For this review, take the finished solid that the model builds, in its own axes (mm). A direction names the side the tool comes from. Coordinates: 2 decimals unless noted, no trailing zeros. Write each loop counter-clockwise with the first axis right and the second up, starting at its lowest first coordinate (ties: lowest second). Pieces come first, ordered by that corner, then holes. Notation, with made-up numbers: M 19,31.25 L 50,31.25 A17 ccw 50,52.25 Z; hole C -3,-5.5 d2. An arc over 180 degrees is marked long. One line per question, with ' | ' between items.
from build123d import *

# Parameters (mm, degrees)
BOSS_EXTRUDE1_DEPTH = 10
BOSS_EXTRUDE2_DEPTH = 10
SKETCH3_R           = 18.5
CUT_EXTRUDE1_DEPTH  = 7
SKETCH4_R           = 14
CUT_EXTRUDE2_DEPTH  = 181.671916356
SKETCH5_R           = 3.5
CUT_EXTRUDE3_DEPTH  = 181.671916356
SKETCH6_R           = 8
CUT_EXTRUDE4_DEPTH  = 5
CUT_EXTRUDE5_DEPTH  = 4


with BuildPart() as part:
    # Sketch1 → Boss-Extrude1 (new body)
    with BuildSketch(Plane(origin=(0, 0, 0), x_dir=(1, 0, 0), z_dir=(0, 1, 0))):
        with BuildLine():
            Line((-50.126401057, 19.839201524), (-7.169705454, -10.239400554))
            ThreePointArc((-7.169705454, -10.239400554), (0, -12.5), (7.169705454, -10.239400554))
            Line((7.169705454, -10.239400554), (50.126401057, 19.839201524))
            ThreePointArc((50.126401057, 19.839201524), (54.194564303, 26.060188175), (52.845996063, 33.369907103))
            ThreePointArc((52.845996063, 33.369907103), (0, 62.5), (-52.845996063, 33.369907103))
            ThreePointArc((-52.845996063, 33.369907103), (-54.194564303, 26.060188175), (-50.126401057, 19.839201524))
        make_face()
    extrude(amount=BOSS_EXTRUDE1_DEPTH)

    # Sketch2 → Boss-Extrude2 (add)
    with BuildSketch(Plane(origin=(0, 0, 0), x_dir=(1, 0, 0), z_dir=(0, 1, 0))):
        with BuildLine():
            Line((-22, 0.144883481), (-22, -150))
            ThreePointArc((-22, -150), (0, -172), (22, -150))
            Line((22, -150), (22, 0.144883481))
            Line((22, 0.144883481), (7.169705454, -10.239400554))
            ThreePointArc((7.169705454, -10.239400554), (0, -12.5), (-7.169705454, -10.239400554))
            Line((-7.169705454, -10.239400554), (-22, 0.144883481))
        make_face()
    extrude(amount=BOSS_EXTRUDE2_DEPTH)

    # Sketch3 → Cut-Extrude1 (cut)
    with BuildSketch(Plane(origin=(0, 10, 0), x_dir=(1, 0, 0), z_dir=(0, 1, 0))):
        with Locations(Location((0, 0, 0), (0, 0, 270))):
            Circle(SKETCH3_R)
    extrude(amount=-CUT_EXTRUDE1_DEPTH, mode=Mode.SUBTRACT)

    # Sketch4 → Cut-Extrude2 (cut, through all)
    with BuildSketch(Plane(origin=(0, 10, 0), x_dir=(1, 0, 0), z_dir=(0, 1, 0))):
        with Locations(Location((0, 0, 0), (0, 0, 270))):
            Circle(SKETCH4_R)
    extrude(amount=-CUT_EXTRUDE2_DEPTH, mode=Mode.SUBTRACT)

    # Sketch5 → Cut-Extrude3 (cut, through all)
    with BuildSketch(Plane(origin=(0, 10, 0), x_dir=(1, 0, 0), z_dir=(0, 1, 0))):
        with Locations(Location((0, -150, 0), (0, 0, 270))):
            Circle(SKETCH5_R)
    extrude(amount=-CUT_EXTRUDE3_DEPTH, mode=Mode.SUBTRACT)

    # Sketch6 → Cut-Extrude4 (cut)
    with BuildSketch(Plane.XZ):
        with Locations(Location((0, 150, 0), (0, 0, 270))):
            Circle(SKETCH6_R)
    extrude(amount=-CUT_EXTRUDE4_DEPTH, mode=Mode.SUBTRACT)

    # Sketch7 → Cut-Extrude5 (cut)
    with BuildSketch(Plane(origin=(0, 10, 0), x_dir=(1, 0, 0), z_dir=(0, 1, 0))):
        Polygon((4.618802154, -150), (2.309401077, -146), (-2.309401077, -146), (-4.618802154, -150), (-2.309401077, -154), (2.309401077, -154), align=None)
    extrude(amount=-CUT_EXTRUDE5_DEPTH, mode=Mode.SUBTRACT)


solid = part.part
1) We need section C-C on z = 110.5. State the section outline as (x, y) points, then the cut area to 3 significant figures.
Responses:
outline: M -22,0 L 22,0 L 22,10 L -22,10 Z | area: 440 mm^2
2) We need section A-A on x = 0. State the section outline as (y, z) points, then the cut area to 3 significant figures.
Responses:
outline: M 0,-62.5 L 10,-62.5 L 10,-18.5 L 3,-18.5 L 3,-14 L 0,-14 Z; M 0,14 L 3,14 L 3,18.5 L 10,18.5 L 10,146 L 6,146 L 6,146.5 L 5,146.5 L 5,142 L 0,142 Z; M 0,158 L 5,158 L 5,153.5 L 6,153.5 L 6,154 L 10,154 L 10,172 L 0,172 Z | area: 1,880 mm^2
3) To check wall thickness, follow line 1 along X through (y, z) = (2.9, 150); line 2 along X through (y, z) = (0.6, 0); line 3 along X through (y, z) = (1.5, 103). State the ranges of each line that lie inside material, in increasing order. Write a range as [from, to].
Responses:
line 1: [-22, -8], [8, 22] | line 2: [-22, -14], [14, 22] | line 3: [-22, 22]
4) The part is to be moulded in two halves that separate along X. For faces 5 (the flat face through (-1, 10, 27)), 6 (the flat face through (-36.26, 4.93, -10.13)), 7 (the cylindrical face through (-7.086, 6.549, 17.089)), say which applies: +X half, -X half, draft (parallel to the pull), parting line (faces both ways), or undercut.
Responses:
face 5: draft | face 6: -X half | face 7: undercut
5) Insertion check: pin 1 Ø5 at (x, y) = (9, 5.5) entering from -Z; pin 2 Ø5 at (y, z) = (3, 52.5) entering from -X; pin 3 Ø8 at (x, z) = (1, 147) entering from -Y. Each pin has a flat end and moves straight along its axis. Give the tip position at first contact, or say it passes through.
Responses:
pin 1: z = -62.16 | pin 2: x = -22 | pin 3: y = 5
6) We need section B-B on y = 7.75. State the section outline as (x, z) points.
Responses:
outline: M -52.85,-33.37 A62.5 ccw 52.85,-33.37 A10 ccw 50.13,-19.84 L 22,-0.14 L 22,150 A22 ccw -22,150 L -22,-0.14 L -50.13,-19.84 A10 ccw Z; hole C 0,0 d37; hole M -4.62,150 L -2.31,146 L 2.31,146 L 4.62,150 L 2.31,154 L -2.31,154 Z
7) Machinability: for faces 1 (the flat face through (22, 5, 76)), 2 (the cylindrical face through (0, 2, 158)), 3 (the flat face through (3.48, 8.03, 148.03)), 4 (the flat face through (-22, 5, 74)), which of the approach directions +Z, -Z, +X, -X, +Y, -Y give a long, thin tool a straight path to every point of the face, cutting with its end or side? Answer none if there is none.
Responses:
face 1: +Z, +X, +Y, -Y | face 2: -Y | face 3: +Y | face 4: +Z, -X, +Y, -Y
